Read the model definition and answer for the solid it produces. Units are mm, in the model's axes. Face numbers are marked on the shaded views. A direction names the side the tool comes from. Give positions to 0.01 mm unless a question says otherwise; leave off trailing zeros. Write each loop counter-clockwise with the first axis right and the second up, starting at its lowest first coordinate (ties: lowest second). Pieces come first, ordered by that corner, then holes. Notation, with made-up numbers: M 79.5,0 L 117.5,0 A24 cw 117.5,14 Z; hole C 10,-24.5 d4. An arc over 180 degrees is marked long. Use a Markdown table: item, result. Add a question column.
Item 1: For the marked faces 4, 5, 6, 7 and 8, determine the directions among +Z, -Z, +X, -X, +Y, -Y from which every point of the face is accessible in a straight line to the end or side of a thin tool.
Item 2: The mould has two halves that part along X. Classify the marked faces 1, 2 and 3: pulls with the +X half, pulls with the -X half, needs draft (parallel to the pull), parting line crosses it, or undercut.
Item 3: Consider probe 1 along X at (y, z) = (1.25, 1.5); probe 2 along X at (y, z) = (6.35, -2.75); probe 3 along Z at (x, y) = (5.25, 6.35). Determine where each line is inside the solid, lowest interval first. Write a range as [from, to].
Item 4: Given P1, Ø3.5, axis at x = -3.175, y = 6.35, coming from the -Z side; P2, Ø6.5, axis at x = -11, y = 5.5, coming from the -Z side (3 decimals); P3, Ø2, axis at x = -25.5, y = 5.5, coming from the -Z side; P4, Ø7, axis at y = 7.5, z = 2, coming from the -X side, each flat-ended and moving along its own axis, determine where each tip first touches the part or whether it passes through.
Item 5: A cutting plane is placed at B-B on z = 12. Determine the outline of the cut face in (x, y).
Item 6: A cutting plane is placed at C-C on z = -11.5. Determine the outline of the cut face in (x, y), then the cut area to 3 significant figures.
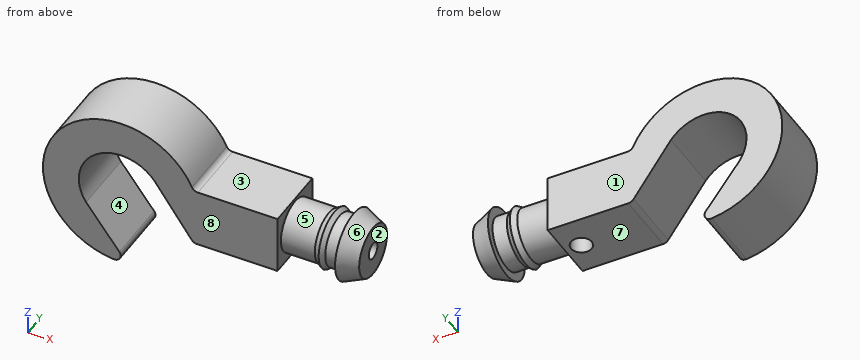
from build123d import *

# Parameters (mm, degrees)
SKETCH2_W                            = 15.24
SKETCH2_H                            = 11.43
BOSS_EXTRUDE2_DEPTH                  = 12.7
F_10_32_TAPPED_HOLE1_D               = 4.0386
F_10_32_TAPPED_HOLE1_DEPTH           = 7.112
F_10_32_TAPPED_HOLE1_TIP             = 1.213317848
F_1_8_START                          = -1.927032922
F_1_8_0_125_DIAMETER_HOLE1_OUTLINE_R = 1.5875
F_1_8_0_125_DIAMETER_HOLE1_DEPTH     = 17.167008702
F_1_8_0_125_DIAMETER_HOLE1_2_ANGLE   = 43.851778
BOSS_EXTRUDE4_DEPTH                  = 12.7
FILLET3_R                            = 1.27


with BuildPart() as part:
    # Sketch2 → Boss-Extrude2 (new body)
    with BuildSketch(Plane(origin=(0, 0, 0), x_dir=(1, 0, 0), z_dir=(0, 1, 0))):
        with Locations((-7.62, 0)):
            Rectangle(SKETCH2_W, SKETCH2_H)
    extrude(amount=BOSS_EXTRUDE2_DEPTH)

    # #10-32 Tapped Hole1
    with Locations(Plane(origin=(0, 0, -5.715), x_dir=(-1, 0, 0), z_dir=(0, 0, -1))):
        with Locations((3.175, 6.35)):
            Hole(F_10_32_TAPPED_HOLE1_D / 2, depth=F_10_32_TAPPED_HOLE1_DEPTH)
            with Locations((0, 0, -(F_10_32_TAPPED_HOLE1_DEPTH + F_10_32_TAPPED_HOLE1_TIP / 2))):  # 118° drill point
                Cone(0, F_10_32_TAPPED_HOLE1_D / 2, F_10_32_TAPPED_HOLE1_TIP, mode=Mode.SUBTRACT)

    # Sketch3 → Revolve1 (revolve)
    with BuildSketch(Plane.XY):
        Polygon((0, 6.35), (0, 11.457170435), (3.81, 11.457170435), (6.60398789, 11.457170435), (7.698956629, 12.092170435), (8.63598789, 11.457170435), (11.42997578, 11.457170435), (11.42997578, 13.108170435), (15.23997578, 11.43), (15.23997578, 6.35), align=None)
    revolve(axis=Axis((15.23997578, 6.35, 0), (-1, 0, 0)))

    # 1/8 (0.125) Diameter Hole1: read off the stored shape, not the designer's step
    # 1/8 (0.125) Diameter Hole1 outline → 1/8 (0.125) Diameter Hole1 (cut)
    with BuildSketch(Plane.YZ.offset(F_1_8_START)):
        with Locations((6.35, 0)):
            Circle(F_1_8_0_125_DIAMETER_HOLE1_OUTLINE_R)
    extrude(amount=F_1_8_0_125_DIAMETER_HOLE1_DEPTH, mode=Mode.SUBTRACT)

    # 1_8 _0.125_ Diameter Hole1 2 outline → 1_8 _0.125_ Diameter Hole1 2 (revolve)
    with BuildSketch(Plane(origin=(-3.175, 6.35, 0), x_dir=(0.9276676260373513, -0.3734069838691089, 0), z_dir=(-0.3734069838691089, -0.9276676260373513, 0))):
        Polygon((2.0193, 1.587640849), (1.702020347, 1.587640849), (2.0193, 1.397), align=None)
    revolve(axis=Axis((-3.175, 6.35, 0), (0, 0, 1)), revolution_arc=F_1_8_0_125_DIAMETER_HOLE1_2_ANGLE)

    # Sketch12 → Boss-Extrude4 (add)
    with BuildSketch(Plane(origin=(0, 0, 0), x_dir=(1, 0, 0), z_dir=(0, 1, 0))):
        with BuildLine():
            Line((-15.24, 5.715), (-16.352141882, 5.715))
            Line((-16.352141882, 5.715), (-23.999818432, -5.113929199))
            ThreePointArc((-23.999818432, -5.113929199), (-35.367933104, -6.652302982), (-37.296546478, 4.656148527))
            Line((-37.296546478, 4.656148527), (-29.247375355, 15.190070325))
            ThreePointArc((-29.247375355, 15.190070325), (-43.450797932, -8.001), (-16.352141882, -5.715))
            Line((-16.352141882, -5.715), (-15.24, -5.715))
            Line((-15.24, -5.715), (-15.24, 5.715))
        make_face()
    extrude(amount=BOSS_EXTRUDE4_DEPTH)

    # Fillet3
    fillet3_edges = [part.edges().sort_by_distance(p)[0] for p in [
        (-29.247375355, 6.35, -15.190070325),
        (-16.352141882, 6.35, 5.715),
        (-16.352141882, 6.35, -5.715),
    ]]
    fillet(fillet3_edges, radius=FILLET3_R)


solid = part.part
Filled in:
| question | item | result |
|---|---|---|
| 1 | face 4 | +Y, -Y |
| 1 | face 5 | none |
| 1 | face 6 | +X |
| 1 | face 7 | -Z, +Y, -Y |
| 1 | face 8 | +Z, -Z, -X, -Y |
| 2 | face 1 | needs draft |
| 2 | face 2 | pulls with the +X half |
| 2 | face 3 | undercut |
| 3 | probe 1 | [-45.65, -38.6], [-21.45, 0], [6.96, 8.33], [11.43, 14.7] |
| 3 | probe 2 | [-45.47, -38.26], [-18.45, -5.19], [-1.16, 15.24] |
| 3 | probe 3 | [-5.11, -1.59], [1.59, 5.11] |
| 4 | P1 | z = 1.56 |
| 4 | P2 | z = -5.715 |
| 4 | P3 | z = 5.69 |
| 4 | P4 | x = -45.72 |
| 5 | outline | M -39.87,0 L -21.09,0 L -21.09,12.7 L -39.87,12.7 Z |
| 6 | outline | M -40.48,0 L -32.07,0 L -32.07,12.7 L -40.48,12.7 Z |
| 6 | area | 107 mm² |
